Autodesk Inventor part; units mm, degrees
ref_plane "YZ Plane" through (0, 0, 0) normal (1, 0, 0) x (0, 1, 0)
ref_plane "XZ Plane" through (0, 0, 0) normal (0, 1, 0) x (-1, 0, 0)
ref_plane "XY Plane" through (0, 0, 0) normal (0, 0, 1) x (1, 0, 0)
sketch "Sketch1" plane through (0, 0, 0) normal (0, 0, 1) x (1, 0, 0)
  line L0 (37, -24.5) -> (-37, -24.5)
  line L1 (-37, -24.5) -> (-37, 24.5)
  line L2 (-37, 24.5) -> (37, 24.5)
  line L3 (37, 24.5) -> (37, -24.5)
  line L4 (37, -24.5) -> (-37, 24.5) construction
  line L5 (-37, -24.5) -> (37, 24.5) construction
  circle A0 centre (0, 0) radius 12.5
  line L6 (-19.05, 19.05) -> (19.05, 19.05)
  line L7 (19.05, 19.05) -> (19.05, -19.05)
  line L8 (19.05, -19.05) -> (-19.05, -19.05)
  line L9 (-19.05, -19.05) -> (-19.05, 19.05)
  line L10 (-19.05, 19.05) -> (19.05, -19.05) construction
  line L11 (19.05, 19.05) -> (-19.05, -19.05) construction
  line L12 (19.05, 19.05) -> (16.9012, 19.05)
  line L13 (16.9012, 19.05) -> (16.9012, 16.9012)
  line L14 (16.9012, 16.9012) -> (19.05, 16.9012)
  line L15 (19.05, 16.9012) -> (19.05, 19.05)
  line L16 (0, 19.05) -> (0, -19.05)
  line L17 (-19.05, 0) -> (19.05, 0)
  line L18 (-16.9012, 19.05) -> (-16.9012, 16.9012)
  line L19 (-16.9012, 16.9012) -> (-19.05, 16.9012)
  line L20 (19.05, 0) -> (-19.05, 0)
  line L21 (16.9012, -19.05) -> (16.9012, -16.9012)
  line L22 (16.9012, -16.9012) -> (19.05, -16.9012)
  line L23 (-16.9012, -16.9012) -> (-19.05, -16.9012)
  line L24 (-16.9012, -19.05) -> (-16.9012, -16.9012)
  line L25 (19.05, 0) -> (30.8356, 0)
  line L26 (-19.05, 0) -> (-30.8356, 0)
  circle A1 centre (-16.9012, 16.9012) radius 2
  circle A2 centre (16.9012, 16.9012) radius 2
  circle A3 centre (16.9012, -16.9012) radius 2
  circle A4 centre (-16.9012, -16.9012) radius 2
  circle A5 centre (-30.8356, 0) radius 2.85
  circle A6 centre (30.8356, 0) radius 2.85
  line L27 (-30.8356, 14.9012) -> (-30.8356, 2.85)
  line L28 (-38.1003, 8.8756) -> (-19.0503, 8.8756)
  line L29 (-22.8548, 8.8756) -> (-20.3098, 8.8756)
  line L30 (-21.4103, 8.8756) -> (-21.4103, 0.9356)
  line L31 (-38.1719, 10.7443) -> (-35.8119, 10.7443)
  line L32 (-35.7403, 8.8756) -> (-35.7403, 16.8156)
  line L33 (-38.1719, 16.29) -> (-38.1719, 13.7)
  line L34 (-35.7403, 14.2256) -> (-19.0503, 14.2256)
  line L35 (-19.0503, 14.2256) -> (-19.0503, 8.8756)
  line L36 (-25.2148, 0.9356) -> (-25.2148, 3.5256)
  line L37 (-21.4103, 3.5256) -> (-38.1003, 3.5256)
  line L38 (-38.1003, 14.2256) -> (-35.7403, 14.2256)
  line L39 (-21.4103, 3.5256) -> (-19.0503, 3.5256)
  line L40 (-19.0503, 3.5256) -> (-19.0503, 8.8756)
  line L41 (-35.8119, 14.2256) -> (-35.8119, 19.0506)
  line L42 (-38.1003, 19.0506) -> (-33.3803, 19.0506)
  line L43 (-33.3803, 19.0506) -> (-33.3803, 14.2256)
  line L44 (-19.0503, 3.5256) -> (-19.0503, -1.2994)
  line L45 (-19.0503, -1.2994) -> (-23.7703, -1.2994)
  line L46 (-23.7703, -1.2994) -> (-23.7703, 3.5256)
  circle A7 centre (-35.7403, 16.8156) radius 1.195
  circle A8 centre (-21.4103, 0.9356) radius 1.195
  line L47 (30.8356, -2.85) -> (30.8356, -14.9012)
  line L48 (33.9356, -8.8756) -> (40.1, -8.8756)
  line L49 (19.05, -8.8756) -> (38.1, -8.8756)
  line L50 (35.74, -8.8756) -> (35.74, -16.8156)
  line L51 (21.41, -8.8756) -> (21.41, -0.9356)
  line L52 (21.41, -3.5256) -> (38.1, -3.5256)
  line L53 (38.1, -3.5256) -> (38.1, -8.8756)
  line L54 (35.74, -14.2256) -> (19.05, -14.2256)
  line L55 (19.05, -3.5256) -> (21.41, -3.5256)
  line L56 (30.8356, -14.2256) -> (33.1956, -14.2256)
  line L57 (38.1, -14.2256) -> (38.1, -8.8756)
  line L58 (19.05, 1.2994) -> (23.77, 1.2994)
  line L59 (23.77, 1.2994) -> (23.77, -3.5256)
  line L60 (38.1, -14.2256) -> (38.1, -19.0506)
  line L61 (38.1, -19.0506) -> (33.38, -19.0506)
  line L62 (33.38, -19.0506) -> (33.38, -14.2256)
  circle A9 centre (21.41, -0.9356) radius 1.195
  circle A10 centre (35.74, -16.8156) radius 1.195
  line L63 (-38.1, -13.7) -> (-19.05, -13.7)
  line L64 (-21.41, -13.7) -> (-21.41, -21.64)
  line L65 (-35.74, -13.7) -> (-35.74, -5.76)
  line L66 (-35.74, -8.35) -> (-19.05, -8.35)
  line L67 (-19.05, -7.985) -> (-19.05, -13.335)
  line L68 (-21.41, -19.05) -> (-38.1, -19.05)
  line L69 (-38.1, -8.35) -> (-35.74, -8.35)
  line L70 (-21.41, -19.05) -> (-19.05, -19.05)
  line L71 (-19.05, -18.685) -> (-19.05, -13.335)
  line L72 (-38.1, -3.525) -> (-33.38, -3.525)
  line L73 (-33.38, -3.525) -> (-33.38, -8.35)
  line L74 (-19.05, -19.05) -> (-19.05, -23.875)
  line L75 (-19.05, -23.875) -> (-23.77, -23.875)
  line L76 (-23.77, -23.875) -> (-23.77, -19.05)
  circle A11 centre (-35.74, -5.76) radius 1.195
  circle A12 centre (-21.41, -21.64) radius 1.195
  line L77 (19.05, 13.7) -> (38.1, 13.7)
  line L78 (35.74, 13.7) -> (35.74, 5.76)
  line L79 (21.41, 13.7) -> (21.41, 21.64)
  line L80 (21.41, 19.05) -> (38.1, 19.05)
  line L81 (38.1, 19.05) -> (38.1, 13.7)
  line L82 (35.74, 8.35) -> (19.05, 8.35)
  line L83 (19.05, 19.05) -> (21.41, 19.05)
  line L84 (35.74, 8.35) -> (38.1, 8.35)
  line L85 (38.1, 8.35) -> (38.1, 13.7)
  line L86 (19.05, 23.875) -> (23.77, 23.875)
  line L87 (23.77, 23.875) -> (23.77, 19.05)
  line L88 (38.1, 8.35) -> (38.1, 3.525)
  line L89 (38.1, 3.525) -> (33.38, 3.525)
  line L90 (33.38, 3.525) -> (33.38, 8.35)
  circle A13 centre (21.41, 21.64) radius 1.195
  circle A14 centre (35.74, 5.76) radius 1.195
  arc A15 (-37, 21.2315) -> (-36.9905, 20.9193) centre (-31.8628, 21.2315) ccw
  line L91 (-38.1, -3.525) -> (-38.1, -19.05)
  line L92 (19.05, 1.2994) -> (19.05, -14.2256)
  circle A16 centre (0, 19.05) radius 2.84
  dimension "d29" = 5.7
  dimension "d0" = 74
  dimension "d1" = 49
  dimension "d2" = 25
  dimension "d3" = 38.1
  dimension "d4" = 38.1
  dimension "d5" = 2.1488
  dimension "d6" = 2.1488
  dimension "d7" = 11.7856
  dimension "d24" = 4
  dimension "d25" = 4
  dimension "d26" = 4
  dimension "d27" = 4
  dimension "d28" = 5.7
  dimension "d30" = 19.05
  dimension "d31" = 2.545
  dimension "d32" = 7.94
  dimension "d33" = 2.36
  dimension "d34" = 7.94
  dimension "d35" = 2.59
  dimension "d36" = 2.59
  dimension "d37" = 4.825
  dimension "d39" = 4.825
  dimension "d40" = 4.72
  dimension "d41" = 2.39
  dimension "d42" = 2.39
  dimension "d43" = 19.05
  dimension "d44" = 2.36
  dimension "d45" = 7.94
  dimension "d46" = 2.36
  dimension "d47" = 7.94
  dimension "d48" = 2.59
  dimension "d49" = 2.59
  dimension "d50" = 4.825
  dimension "d51" = 4.72
  dimension "d52" = 4.825
  dimension "d53" = 4.72
  dimension "d54" = 2.39
  dimension "d55" = 2.39
  dimension "d56" = 19.05
  dimension "d57" = 2.36
  dimension "d58" = 7.94
  dimension "d59" = 2.36
  dimension "d60" = 7.94
  dimension "d61" = 2.59
  dimension "d62" = 2.59
  dimension "d63" = 4.825
  dimension "d64" = 4.72
  dimension "d65" = 4.825
  dimension "d66" = 4.72
  dimension "d67" = 2.39
  dimension "d68" = 2.39
  dimension "d69" = 19.05
  dimension "d70" = 2.36
  dimension "d71" = 7.94
  dimension "d72" = 2.36
  dimension "d73" = 7.94
  dimension "d74" = 2.59
  dimension "d75" = 2.59
  dimension "d76" = 4.825
  dimension "d77" = 4.72
  dimension "d78" = 4.825
  dimension "d79" = 4.72
  dimension "d80" = 2.39
  dimension "d81" = 2.39
extrude "Extrusion1" add sketch "Sketch1" along normal blind 6 contours L0 L1 L68 L76 L75 L74 L8 L7 L54 L62 L61 L3 | A10 | L61 L62 L54 L50 L48 L3 | L1 L63 L64 L68 | L48 L49 L47 L52 L3 | L1 L69 L65 L63 | A12 | L68 L70 L74 L75 L76 | L52 L47 A6 L25 L59 L58 L7 L82 L90 L89 L3 | L50 L54 L47 L49 L48 | A11 | L1 L72 L73 L66 L69 | L65 L66 L9 L63 | L64 L63 L9 L70 | A14 | L89 L90 L82 L84 L3 | L52 L59 L25 A6 L47 | L47 L49 L51 L52 | L1 L37 L27 A5 L26 L46 L45 L9 L66 L73 L72 | L9 L23 A4 L24 L8 | L84 L78 L77 L3 | A6 | L47 L54 L7 L49 | L52 L51 A9 L25 L59 | L1 L28 L27 L37 | L9 L17 A0 L16 L8 L24 A4 L23 | L77 L79 L80 L3 | L82 L7 L77 L78 | L49 L7 L55 L51 | L55 L7 L25 A9 L51 | L25 A9 L7 L58 L59 | L7 L22 A3 L21 L8 L16 A0 L17 | L1 L38 L32 L28 | L37 L46 L26 A5 L27 | L27 L28 L30 L37 | A4 L23 L24 | L24 L23 A4 | A13 | L80 L83 L6 A16 L9 L34 L43 L42 L1 L2 L3 | L7 L17 A0 L16 A16 L6 L13 A2 L14 | A9 L25 | L25 A9 | L7 L8 L21 A3 L22 | L32 L34 L27 L28 | L27 L34 L9 L28 | A5 | L77 L7 L83 L79 | A3 L21 L22 | L22 L21 A3 | L1 L42 L41 A7 L38 | L38 L41 A7 L32 | L32 A7 L41 L42 L43 L34 | L37 L30 A8 L26 L46 | L45 L46 L26 A8 L9 | L17 L9 L19 A1 L18 L6 A16 L16 A0 | L14 A2 L13 L6 L7 | A7 L41 | L28 L9 L39 L30 | L39 L9 L26 A8 L30 | A2 L13 L14 | L14 L13 A2 | A7 L41 | L9 L6 L18 A1 L19 | A8 L26 | L26 A8 | A16 L6 L16 | L16 L6 A16 | A1 L18 L19 | L19 L18 A1 | L6 A16
hole "Hole1" at (-16.9012, -16.9012, 0) at (16.9012, -16.9012, 0) at (16.9012, 16.9012, 0) at (-16.9012, 16.9012, 0) direction (0, 0, 1) diameter 1.567 end through all
hole "Hole2" at (-30.8356, 0, 0) at (30.8356, 0, 0) direction (0, 0, 1) diameter 3.4 end through all
hole "Hole3" at (-35.7403, 16.8156, 0) at (-21.4103, 0.9356, 0) at (-35.74, -5.76, 0) at (-21.41, -21.64, 0) at (35.74, -16.8156, 0) at (21.41, -0.9356, 0) at (35.74, 5.76, 0) at (21.41, 21.64, 0) direction (0, 0, 1) diameter 1.567 end through all
hole "Hole4" at (0, 19.05, 0) direction (0, 0, 1) diameter 2.459 end through all
properties part number "adapter-plate"
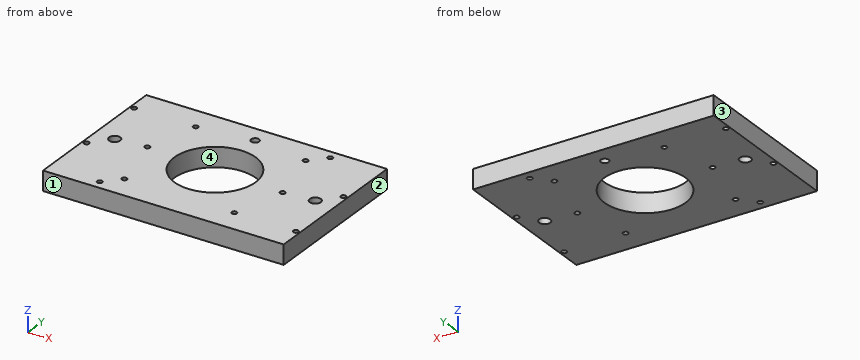
Here's how the part is built. I have some questions about the finished solid (model axes, mm). Face numbers are marked on the shaded views. Round coordinates to 2 decimals unless told otherwise and drop trailing zeros. Write each loop counter-clockwise with the first axis right and the second up, starting at its lowest first coordinate (ties: lowest second). Pieces come first, ordered by that corner, then holes. Notation, with made-up numbers: (-2.5, -16.5) -> (15.5, -16.5) arc R13 cw to (15.5, 3.5) -> close; hole circle Ø7 at (56, -4.5). An arc over 180 degrees is marked (long way). One line per item, written item: value.
1) If I drill on line 1 (Y direction, x = -17, z = 3.4); line 2 (X direction, y = 0, z = 3.85); line 3 (Y direction, x = -35.74, z = 3.15), over which ranges is the centre line in solid material (lowest first)? Write a range as [from, to].
Filled sheet:
line 1: y = [-24.5, -17.68], [-16.12, 16.12], [17.68, 24.5]
line 2: x = [-37, -32.54], [-29.14, -12.5], [12.5, 29.14], [32.54, 37]
line 3: y = [-24.5, -6.54], [-4.98, 16.03], [17.6, 24.5]
2) Suppose I cut it at B-B on x = 21.41. List the corners of the cut face in (y, z) for me, plus the area to 3 significant figures.
Filled sheet:
outline: (-24.5, 0) -> (-1.72, 0) -> (-1.72, 6) -> (-24.5, 6) -> close; (-0.15, 0) -> (20.86, 0) -> (20.86, 6) -> (-0.15, 6) -> close; (22.42, 0) -> (24.5, 0) -> (24.5, 6) -> (22.42, 6) -> close
area: 275 mm2
3) Suppose I cut it at C-C on z = 2.65. Give the number of separate pieces and of enclosed holes in the cut face, plus the area to 3 significant figures.
Filled sheet:
separate pieces: 1
enclosed holes: 16
area: 3,090 mm2
4) We'd pull the mould along X, two halves only. Please class the marked faces 1, 2, 3 and 4: released by +X, released by -X, zero draft, split by the parting line, or undercut.
Filled sheet:
face 1: zero draft
face 2: released by +X
face 3: released by -X
face 4: undercut
5) Suppose I cut it at D-D on y = -11. List the corners of the cut face in (x, z) for me.
Filled sheet:
outline: (-37, 0) -> (-5.94, 0) -> (-5.94, 6) -> (-37, 6) -> close; (5.94, 0) -> (37, 0) -> (37, 6) -> (5.94, 6) -> close
6) Suppose I cut it at A-A on y = 19.05. List the corners of the cut face in (x, z) for me.
Filled sheet:
outline: (-37, 0) -> (-1.23, 0) -> (-1.23, 6) -> (-37, 6) -> close; (1.23, 0) -> (37, 0) -> (37, 6) -> (1.23, 6) -> close
